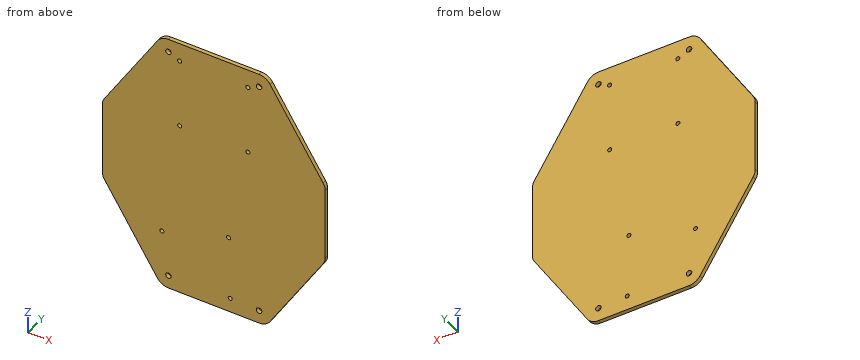
from build123d import *

# Parameters (mm, degrees)
SKETCH_1_R      = 1.55
SKETCH_1_R_2    = 2.1
EXTRUDE_1_DEPTH = 3


with BuildPart() as part:
    # 草图1 → 凸台-拉伸1 (new body)
    with BuildSketch(Plane(origin=(0, 0, 0), x_dir=(1, 0, 0), z_dir=(0, 1, 0))):
        with BuildLine():
            Line((-85, 32.937018863), (-85, 87.062981137))
            ThreePointArc((-85, 87.062981137), (-84.594734169, 89.880972661), (-83.411784754, 92.47055705))
            Line((-83.411784754, 92.47055705), (-42.952272627, 155.407575913))
            ThreePointArc((-42.952272627, 155.407575913), (-39.332368552, 158.777122511), (-34.540487874, 160))
            Line((-34.540487874, 160), (34.540487874, 160))
            ThreePointArc((34.540487874, 160), (39.332368552, 158.777122511), (42.952272627, 155.407575913))
            Line((42.952272627, 155.407575913), (83.411784754, 92.47055705))
            ThreePointArc((83.411784754, 92.47055705), (84.594734169, 89.880972661), (85, 87.062981137))
            Line((85, 87.062981137), (85, 32.937018863))
            ThreePointArc((85, 32.937018863), (84.594734169, 30.119027339), (83.411784754, 27.52944295))
            Line((83.411784754, 27.52944295), (42.952272627, -35.407575913))
            ThreePointArc((42.952272627, -35.407575913), (39.332368552, -38.777122511), (34.540487874, -40))
            Line((34.540487874, -40), (-34.540487874, -40))
            ThreePointArc((-34.540487874, -40), (-39.332368552, -38.777122511), (-42.952272627, -35.407575913))
            Line((-42.952272627, -35.407575913), (-83.411784754, 27.52944295))
            ThreePointArc((-83.411784754, 27.52944295), (-84.594734169, 30.119027339), (-85, 32.937018863))
        make_face()
        with Locations(Location((-26, 26, 0), (0, 0, 270))):
            Circle(SKETCH_1_R, mode=Mode.SUBTRACT)
        with Locations(Location((26, 26, 0), (0, 0, 270))):
            Circle(SKETCH_1_R, mode=Mode.SUBTRACT)
        with Locations(Location((26, -26, 0), (0, 0, 270))):
            Circle(SKETCH_1_R, mode=Mode.SUBTRACT)
        with Locations(Location((-26, -26, 0), (0, 0, 270))):
            Circle(SKETCH_1_R, mode=Mode.SUBTRACT)
        with Locations(Location((-39.5, 116.11, 0), (0, 0, 270))):
            Circle(SKETCH_1_R, mode=Mode.SUBTRACT)
        with Locations(Location((11.3, 100.87, 0), (0, 0, 270))):
            Circle(SKETCH_1_R, mode=Mode.SUBTRACT)
        with Locations(Location((12.57, 149.13, 0), (0, 0, 270))):
            Circle(SKETCH_1_R, mode=Mode.SUBTRACT)
        with Locations(Location((-34.540487874, -30, 0), (0, 0, 270))):
            Circle(SKETCH_1_R_2, mode=Mode.SUBTRACT)
        with Locations(Location((34.540487874, -30, 0), (0, 0, 270))):
            Circle(SKETCH_1_R_2, mode=Mode.SUBTRACT)
        with Locations(Location((34.540487874, 150, 0), (0, 0, 270))):
            Circle(SKETCH_1_R_2, mode=Mode.SUBTRACT)
        with Locations(Location((-34.540487874, 150, 0), (0, 0, 270))):
            Circle(SKETCH_1_R_2, mode=Mode.SUBTRACT)
    extrude(amount=EXTRUDE_1_DEPTH)


solid = part.part
The listing builds one solid part. Answer for the finished solid, in the listing's coordinates (mm). Give positions to 0.01 mm unless a question says otherwise; leave off trailing zeros. Order: outer loops, then holes, each group sorted by start corner. A loop starts at its lowest first (then second) coordinate and runs counter-clockwise, first axis right, second up. Notation, with made-up numbers: (66, 25) - (93, 25) arc R11 ccw to (93, 34) - close; hole circle Ø5 at (-18, 33.25). An arc over 180 degrees is marked (long way). Use one line per item in the form item = value.
1) This flat-tipped pin is pushed along its axis until it touches: pin 1 (3 mm diameter, centred on x = -39.5, z = -116.11, fed in from -Y). Where does it stop, or does it pass through?
Verdict:
pin_1 = through
2) Find section A-A on y = 2.3. Give the number of separate pieces and of enclosed holes in the cut face, and give its area (3 significant figures).
Verdict:
separate_pieces = 1
enclosed_holes = 11
area = 27,600 mm^2
3) Find section B-B on z = -126. Determine the outline of the cut face in (x, y), and give its area (3 significant figures).
Verdict:
outline = (-61.86, 0) - (61.86, 0) - (61.86, 3) - (-61.86, 3) - close
area = 371 mm^2
4) Consider probe 1 along X at (y, z) = (1.7, -150); probe 2 along X at (y, z) = (2.1, -149.13); probe 3 along X at (y, z) = (0.6, 26). Determine where each line is inside the solid, lowest interval first. Write a range as [from, to].
Verdict:
probe_1 = [-46.43, -36.64], [-32.44, 11.29], [13.85, 32.44], [36.64, 46.43]
probe_2 = [-46.99, -36.45], [-32.63, 11.02], [14.12, 32.63], [36.45, 46.99]
probe_3 = [-49, -27.55], [-24.45, 24.45], [27.55, 49]
5) Find section C-C on x = -63. Determine the outline of the cut face in (y, z).
Verdict:
outline = (0, -124.22) - (3, -124.22) - (3, 4.22) - (0, 4.22) - close
